Build history of the part. All positions in model axes, mm. A direction names the side the tool comes from. Give positions to 0.01 mm unless a question says otherwise; leave off trailing zeros.
1) Band-saw the part on A-A on z = 402.5. State how many separate pieces and enclosed holes the cut face has, then the cut area to 3 significant figures.
2) Wall check: line 1 (Y direction, x = 25.5, z = 190); line 2 (Y direction, x = 15, z = 307); line 3 (X direction, y = 25, z = 282.5). Give the ranges that are in metal, low to high.
3) Two-plate mould, pull along X, no slides. Class faces 3 (the cylindrical face through (-19.5, -14.9, 257)), 4 (the flat face through (30, 24, 265)), 5 (the flat face through (0, 27.5, 265)), 6 (the flat face through (11.251, 10.971, 529.978)): +X half, -X half, draft (parallel to the pull), parting line (faces both ways), or undercut.
4) Flat gauge pin, fed straight in: P1, Ø1.8, axis at x = 14, z = 393.5, coming from the -Y side. Where does the tip first touch, or does it go through?
5) 3-axis set-ups, long thin cutter, end or side, ignore diameter. For faces 1 (the flat face through (30, -24, 255)), 2 (the cylindrical face through (-19.5, 15.1, 263.2)): which of +Z, -Z, +X, -X, +Y, -Y reach the whole face in a straight line?
```python
from build123d import *

# Parameters (mm, degrees)
F0_R          = 3
F0_R_2        = 2.5
F1_DEPTH      = 537.86
F2_R          = 2
F3_R          = 7
F5_DEPTH      = 30
F5_DEPTH_BACK = 30


# Not quite as in the source:
# - a feature names something its author has since deleted; it is built from what else it names


with BuildPart() as f1:
    # F0 (on Top) → F1 (new body)
    with BuildSketch(Plane.XY):
        with BuildLine():
            Line((18.15, -30), (30, -30))
            Line((30, -30), (30, -18.15))
            Line((30, -18.15), (27.5, -18.15))
            Line((27.5, -18.15), (27.5, -20.15))
            Line((27.5, -20.15), (21.5477069044, -20.15))
            ThreePointArc((21.5477069044, -20.15), (19.5, -15), (21.5477069044, -9.85))
            Line((21.5477069044, -9.85), (27.5, -9.85))
            Line((27.5, -9.85), (27.5, -11.85))
            Line((27.5, -11.85), (30, -11.85))
            Line((30, -11.85), (30, 11.85))
            Line((30, 11.85), (27.5, 11.85))
            Line((27.5, 11.85), (27.5, 9.85))
            Line((27.5, 9.85), (21.5477069044, 9.85))
            ThreePointArc((21.5477069044, 9.85), (19.5, 15), (21.5477069044, 20.15))
            Line((21.5477069044, 20.15), (27.5, 20.15))
            Line((27.5, 20.15), (27.5, 18.15))
            Line((27.5, 18.15), (30, 18.15))
            Line((30, 18.15), (30, 30))
            Line((30, 30), (18.15, 30))
            Line((18.15, 30), (18.15, 27.5))
            Line((18.15, 27.5), (20.15, 27.5))
            Line((20.15, 27.5), (20.15, 21.5477069044))
            ThreePointArc((20.15, 21.5477069044), (15, 19.5), (9.85, 21.5477069044))
            Line((9.85, 21.5477069044), (9.85, 27.5))
            Line((9.85, 27.5), (11.85, 27.5))
            Line((11.85, 27.5), (11.85, 30))
            Line((11.85, 30), (-11.85, 30))
            Line((-11.85, 30), (-11.85, 27.5))
            Line((-11.85, 27.5), (-9.85, 27.5))
            Line((-9.85, 27.5), (-9.85, 21.5477069044))
            ThreePointArc((-9.85, 21.5477069044), (-15, 19.5), (-20.15, 21.5477069044))
            Line((-20.15, 21.5477069044), (-20.15, 27.5))
            Line((-20.15, 27.5), (-18.15, 27.5))
            Line((-18.15, 27.5), (-18.15, 30))
            Line((-18.15, 30), (-30, 30))
            Line((-30, 30), (-30, 18.15))
            Line((-30, 18.15), (-27.5, 18.15))
            Line((-27.5, 18.15), (-27.5, 20.15))
            Line((-27.5, 20.15), (-21.5477069044, 20.15))
            ThreePointArc((-21.5477069044, 20.15), (-19.5, 15), (-21.5477069044, 9.85))
            Line((-21.5477069044, 9.85), (-27.5, 9.85))
            Line((-27.5, 9.85), (-27.5, 11.85))
            Line((-27.5, 11.85), (-30, 11.85))
            Line((-30, 11.85), (-30, -11.85))
            Line((-30, -11.85), (-27.5, -11.85))
            Line((-27.5, -11.85), (-27.5, -9.85))
            Line((-27.5, -9.85), (-21.5477069044, -9.85))
            ThreePointArc((-21.5477069044, -9.85), (-19.5, -15), (-21.5477069044, -20.15))
            Line((-21.5477069044, -20.15), (-27.5, -20.15))
            Line((-27.5, -20.15), (-27.5, -18.15))
            Line((-27.5, -18.15), (-30, -18.15))
            Line((-30, -18.15), (-30, -30))
            Line((-30, -30), (-18.15, -30))
            Line((-18.15, -30), (-18.15, -27.5))
            Line((-18.15, -27.5), (-20.15, -27.5))
            Line((-20.15, -27.5), (-20.15, -21.5477069044))
            ThreePointArc((-20.15, -21.5477069044), (-15, -19.5), (-9.85, -21.5477069044))
            Line((-9.85, -21.5477069044), (-9.85, -27.5))
            Line((-9.85, -27.5), (-11.85, -27.5))
            Line((-11.85, -27.5), (-11.85, -30))
            Line((-11.85, -30), (11.85, -30))
            Line((11.85, -30), (11.85, -27.5))
            Line((11.85, -27.5), (9.85, -27.5))
            Line((9.85, -27.5), (9.85, -21.5477069044))
            ThreePointArc((9.85, -21.5477069044), (15, -19.5), (20.15, -21.5477069044))
            Line((20.15, -21.5477069044), (20.15, -27.5))
            Line((20.15, -27.5), (18.15, -27.5))
            Line((18.15, -27.5), (18.15, -30))
        make_face()
        with Locations((-25, -25)):
            Circle(F0_R, mode=Mode.SUBTRACT)
        with Locations((-15, -15)):
            Circle(F0_R_2, mode=Mode.SUBTRACT)
        with Locations((25, -25)):
            Circle(F0_R, mode=Mode.SUBTRACT)
        with Locations((15, -15)):
            Circle(F0_R_2, mode=Mode.SUBTRACT)
        with Locations((-25, 25)):
            Circle(F0_R, mode=Mode.SUBTRACT)
        with Locations((-15, 15)):
            Circle(F0_R_2, mode=Mode.SUBTRACT)
        Polygon((-7, 22), (-7, 27.5), (0, 27.5), (7, 27.5), (7, 22), (10, 16), (10, 10), (16, 10), (22, 7), (27.5, 7), (27.5, 0), (27.5, -7), (22, -7), (16, -10), (10, -10), (10, -16), (7, -22), (7, -27.5), (0, -27.5), (-7, -27.5), (-7, -22), (-10, -16), (-10, -10), (-16, -10), (-22, -7), (-27.5, -7), (-27.5, 0), (-27.5, 7), (-22, 7), (-16, 10), (-10, 10), (-10, 16), align=None, mode=Mode.SUBTRACT)
        with Locations((15, 15)):
            Circle(F0_R_2, mode=Mode.SUBTRACT)
        with Locations((25, 25)):
            Circle(F0_R, mode=Mode.SUBTRACT)
    extrude(amount=F1_DEPTH)

    # F2
    f2_edges = [f1.edges().sort_by_distance(p)[0] for p in [
        (-7, 27.5, 268.93),
        (7, 27.5, 268.93),
    ]]
    fillet(f2_edges, radius=F2_R)

    # F3
    f3_edges = [f1.edges().sort_by_distance(p)[0] for p in [
        (-10, 16, 268.93),
        (10, 16, 268.93),
    ]]
    fillet(f3_edges, radius=F3_R)

    # F4 (on Right) → F5 (cut, two sides)
    with BuildSketch(Plane.YZ) as f5_sk:
        Polygon((-77.6874923482, 797.8406045251), (-234.1260457354, 733.041634034), (-126.4385533872, 473.061029509), (30, 537.86), align=None)
    extrude(amount=F5_DEPTH, mode=Mode.SUBTRACT)
    extrude(f5_sk.sketch, amount=-F5_DEPTH_BACK, mode=Mode.SUBTRACT)


solid = f1.part
```
Findings below:
1. separate pieces: 1
1. enclosed holes: 9
1. area: 1,080 mm2
2. line 1: y = -30 to -27.96, -22.04 to -20.15, -9.85 to -7, 7 to 9.85, 20.15 to 22.04, 27.96 to 30
2. line 2: y = -19.5 to -17.5, -12.5 to -10, 10 to 12.5, 17.5 to 19.5
2. line 3: x = -30 to -28, -22 to -20.15, -9.85 to -7, 7 to 9.85, 20.15 to 22, 28 to 30
3. face 3: undercut
3. face 4: +X half
3. face 5: undercut
3. face 6: draft
4. P1: stops at y = -19.74
5. face 1: +Z, -Z, +X, +Y, -Y
5. face 2: +Z, -Z
